Can you work these out from the model? Positions are in its coordinate system, mm. A direction names the side the tool comes from. Round coordinates to 2 decimals unless told otherwise and drop trailing zeros. Write each loop counter-clockwise with the first axis right and the second up, starting at its lowest first coordinate (ties: lowest second). Pieces come first, ordered by that corner, then holes. Notation, with made-up numbers: M -38,32.25 L 20,32.25 A18 ccw 20,47.25 Z; hole C 14,37 d6. An arc over 180 degrees is marked long. Answer in a Markdown table with one row per item. Add a question column.
(1) For faces 4 (the face through (-1, -37.6, 22)), 5 (the face through (-1, 1, 0)), which set-ups out of +Z, -Z, +X, -X, +Y, -Y let a thin tool reach every point of the face, with its end or its side?
(2) Suppose I cut it at C-C, the plane x = 24. Write out the boundary of the cut face in (y, z), then the cut area to 3 significant figures.
(3) Suppose I cut it at A-A, the plane z = 16. Write out the boundary of the cut face in (x, y), then the cut area to 3 significant figures.
(4) If we mould it in two halves opening along X, with no side actions, what happens to faces 1 (the face through (-1, 37.6, 22)), 2 (the face through (-62.5, -1, 20)), 3 (the face through (-19, -38, 40))? For each: released by +X, released by -X, zero draft, split by the parting line, or undercut.
(5) I'm going to push a flat-ended pin straight in: pin 1 (5 mm diameter, centred on x = -9, y = 23.5, fed in from +Z). Where does the tip first touch, or does it pass through?
(6) Suppose I cut it at B-B, the plane y = -3.5. Write out the boundary of the cut face in (x, z), then the cut area to 3 significant figures.
(7) If I drill on probe 1 along X at (y, z) = (15, 25); probe 2 along Y at (x, z) = (-15.5, 14.5); probe 3 along Z at (x, y) = (-44.5, -29), over which ranges is the centre line in solid material (lowest first)?
from build123d import *

# Parameters (mm, degrees)
SKETCH_1_W          = 125
SKETCH_1_H          = 80
EXTRUDE_1_DEPTH     = 40
SKETCH_2_W          = 120.2
SKETCH_2_H          = 75.2
CUT_EXTRUDE_1_DEPTH = 37.6
FILLET_1_R          = 1
FILLET_2_R          = 1


with BuildPart() as part:
    # Эскиз1 → Бобышка-Вытянуть1 (new body)
    with BuildSketch(Plane.XY):
        Rectangle(SKETCH_1_W, SKETCH_1_H)
    extrude(amount=EXTRUDE_1_DEPTH)

    # Эскиз2 → Вырез-Вытянуть1 (cut)
    with BuildSketch(Plane.XY.offset(40)):
        Rectangle(SKETCH_2_W, SKETCH_2_H)
    extrude(amount=-CUT_EXTRUDE_1_DEPTH, mode=Mode.SUBTRACT)

    # Скругление1
    fillet_1_edges = [part.edges().sort_by_distance(p)[0] for p in [
        (0, -40, 0),
        (-62.5, 0, 0),
        (0, 40, 0),
        (62.5, 0, 0),
        (62.5, -40, 20),
        (-62.5, -40, 20),
        (-62.5, 40, 20),
        (62.5, 40, 20),
    ]]
    fillet(fillet_1_edges, radius=FILLET_1_R)

    # Скругление2
    fillet_2_edges = [part.edges().sort_by_distance(p)[0] for p in [
        (60.1, 0, 2.4),
        (60.1, 37.6, 21.2),
        (0, -37.6, 2.4),
        (60.1, -37.6, 21.2),
        (-60.1, 0, 2.4),
        (-60.1, -37.6, 21.2),
        (0, 37.6, 2.4),
        (-60.1, 37.6, 21.2),
    ]]
    fillet(fillet_2_edges, radius=FILLET_2_R)


solid = part.part
Calculated:
| question | item | result |
|---|---|---|
| 1 | face 4 | +Z |
| 1 | face 5 | -Z, +X, -X, +Y, -Y |
| 2 | outline | M -40,1 A1 ccw -39,0 L 39,0 A1 ccw 40,1 L 40,40 L 37.6,40 L 37.6,3.4 A1 cw 36.6,2.4 L -36.6,2.4 A1 cw -37.6,3.4 L -37.6,40 L -40,40 Z |
| 2 | area | 372 mm² |
| 3 | outline | M -62.5,-39 A1 ccw -61.5,-40 L 61.5,-40 A1 ccw 62.5,-39 L 62.5,39 A1 ccw 61.5,40 L -61.5,40 A1 ccw -62.5,39 Z; hole M -60.1,-36.6 A1 ccw -59.1,-37.6 L 59.1,-37.6 A1 ccw 60.1,-36.6 L 60.1,36.6 A1 ccw 59.1,37.6 L -59.1,37.6 A1 ccw -60.1,36.6 Z |
| 3 | area | 961 mm² |
| 4 | face 1 | undercut |
| 4 | face 2 | released by -X |
| 4 | face 3 | zero draft |
| 5 | pin 1 | z = 2.4 |
| 6 | outline | M -62.5,1 A1 ccw -61.5,0 L 61.5,0 A1 ccw 62.5,1 L 62.5,40 L 60.1,40 L 60.1,3.4 A1 cw 59.1,2.4 L -59.1,2.4 A1 cw -60.1,3.4 L -60.1,40 L -62.5,40 Z |
| 6 | area | 480 mm² |
| 7 | probe 1 | -62.5 to -60.1, 60.1 to 62.5 |
| 7 | probe 2 | -40 to -37.6, 37.6 to 40 |
| 7 | probe 3 | 0 to 2.4 |
